Check sheet for the modelled part. Datum: model origin and axes. Units: mm. Coordinates: 2 decimals unless noted, no trailing zeros. Write each loop counter-clockwise with the first axis right and the second up, starting at its lowest first coordinate (ties: lowest second). Pieces come first, ordered by that corner, then holes. Notation, with made-up numbers: (12.5, -23) -> (26.5, -23) arc R22 ccw to (26.5, 3) -> close; hole circle Ø11 at (71.5, -16.5). An arc over 180 degrees is marked (long way). One line per item, written item: value. Start each with the question number.
1) Draft check along X on faces 1 (the flat face through (0, -5, 0)), 2 (the cylindrical face through (4.715, -4.699, 0.21)), 3 (the cylindrical face through (0, -3, 13)). Enter one of: +X half, -X half, draft (parallel to the pull), parting line (faces both ways), or undercut.
2) Scan lines: line 1 along Z through (x, y) = (0, -3.8); line 2 along X through (y, z) = (-3, 15); line 3 along Z through (x, y) = (-1.25, -2.3). Record each from-to range of solid material in increasing order. Write a range as [from, to].
3) Sectioned sample at C-C on x = -1. Give the number of separate pieces and of enclosed holes in the cut face, plus the area to 3 significant figures.
4) Sectioned sample at A-A on y = -2.8. Enter the section's corners in (x, z).
5) Gauge pin test, flat end, axial feed: P1, Ø3.5, axis at x = 0, z = 15, coming from the +Y side. Record the tip position at first contact, or that the pin passes through.
6) Sectioned sample at B-B on z = -8. Enter the section's corners in (x, y).
```python
from build123d import *

# Parameters (mm, degrees)
F0_W     = 10
F0_H     = 30
F1_DEPTH = 5
F3_D     = 4
F4_R     = 1


# Not quite as in the source:
# - a feature of the source that left no trace in its solid (it failed there, or was rolled back) is left out


with BuildPart() as f1:
    # F0 (on Front) → F1 (new body)
    with BuildSketch(Plane.XZ):
        with BuildLine():
            Line((5, -15), (-5, -15))
            ThreePointArc((-5, -15), (0, -20), (5, -15))
        make_face()
        with BuildLine():
            ThreePointArc((5, 15), (0, 20), (-5, 15))
            Line((-5, 15), (5, 15))
        make_face()
        Rectangle(F0_W, F0_H)
    extrude(amount=F1_DEPTH)

    # F3 (through all)
    with Locations(Plane(origin=(0, 0, 0), x_dir=(1, 0, 0), z_dir=(0, 1, 0))):
        with Locations((0, -15), (0, 15)):
            Hole(F3_D / 2)

    # F4
    f4_edges = [f1.edges().sort_by_distance(p)[0] for p in [
        (5, -5, 0),
        (5, 0, 0),
        (0, 0, -20),
        (0, -5, -20),
        (-5, 0, 0),
        (-5, -5, 0),
        (0, 0, 20),
        (0, -5, 20),
    ]]
    fillet(f4_edges, radius=F4_R)


solid = f1.part
```
Answers:
1. face 1: draft
1. face 2: +X half
1. face 3: undercut
2. line 1: z = [-20, -17], [-13, 13], [17, 20]
2. line 2: x = [-5, -2], [2, 5]
2. line 3: z = [-19.84, -16.56], [-13.44, 13.44], [16.56, 19.84]
3. separate pieces: 3
3. enclosed holes: 0
3. area: 163 mm2
4. outline: (-5, -15) arc R5 ccw to (5, -15) -> (5, 15) arc R5 ccw to (-5, 15) -> close; hole circle Ø4 at (0, -15); hole circle Ø4 at (0, 15)
5. P1: passes through
6. outline: (-5, -4) arc R1 ccw to (-4, -5) -> (4, -5) arc R1 ccw to (5, -4) -> (5, -1) arc R1 ccw to (4, 0) -> (-4, 0) arc R1 ccw to (-5, -1) -> close
